Design review of the part built by this model. Coordinates are the model's own, in mm. A direction names the side the tool comes from. Round coordinates to 2 decimals unless told otherwise and drop trailing zeros. Order: outer loops, then holes, each group sorted by start corner. A loop starts at its lowest first (then second) coordinate and runs counter-clockwise, first axis right, second up. Notation, with made-up numbers: (58.5, -3) - (109.5, -3) arc R6 cw to (109.5, 8) - close; hole circle Ø3 at (54, 48.25). An arc over 180 degrees is marked (long way). Answer as a JSON object with one key per item and string values. Group by question number.
Autodesk Inventor part; units mm, degrees
ref_plane "YZ Plane" through (0, 0, 0) normal (1, 0, 0) x (0, 1, 0)
ref_plane "XZ Plane" through (0, 0, 0) normal (0, 1, 0) x (-1, 0, 0)
ref_plane "XY Plane" through (0, 0, 0) normal (0, 0, 1) x (1, 0, 0)
sketch "Sketch1" plane through (0, 0, 0) normal (1, 0, 0) x (0, 1, 0)
  line L0 (0, 0) -> (21.59, 0)
  line L1 (21.59, 0) -> (21.59, -120.8278)
  line L2 (21.59, -120.8278) -> (0, -120.8278)
  line L3 (0, -120.8278) -> (0, 0)
  dimension "d0" = 21.59
  dimension "d1" = 120.8278
extrude "Extrusion1" add sketch "Sketch1" along normal blind 4.7625
sketch "Sketch2" plane through (0, 21.59, 0) normal (0, 1, 0) x (1, 0, 0)
  line L0 (0, 0) -> (-3.2071, -18.1884)
  line L1 (0, 0) -> (18.469, 0) construction
  line L2 (0, 0) -> (13.0579, -2.3025)
  line L3 (0, 0) -> (13.2594, 0) construction
  dimension "d4" = 100
  dimension "d24" = 10
ref_plane "Work Plane1" through (0, 21.59, 0) normal (-0.9848078, 0, -0.1736482) x (-0.1736482, 0, 0.9848078)
sketch "Sketch3" plane through (0, 21.59, 0) normal (-0.9848078, 0, -0.1736482) x (-0.1736482, 0, 0.9848078)
  line L0 (-0.827, 0) -> (-0.827, -21.59)
  line L1 (-0.827, -21.59) -> (-119.8192, -21.59)
  line L2 (-119.8192, -21.59) -> (-119.8192, 0)
  line L3 (-119.8192, 0) -> (-0.827, 0)
  line L4 (0, -21.59) -> (0, 0)
  line L5 (0, -21.59) -> (-0.827, -21.59)
  line L6 (-0.827, 0) -> (-0.827, -21.59)
  line L7 (0, 0) -> (-0.827, 0)
  line L8 (0, -21.59) -> (0, 0)
  circle A0 centre (-0.8636, -10.795) radius 9.525
  dimension "d6" = 21.59
  dimension "d50" = 19.05
  dimension "d51" = 0.8636
extrude "Extrusion2" add sketch "Sketch3" against normal blind 4.7625 contours A0 L4 L0 | L0 A0 | A0 L4
ref_plane "Work Plane3" through (0, 0, 0) normal (-0.1736482, 0, 0.9848078) x (0, 1, 0)
sketch "Sketch9" plane through (4.7625, 0, 0) normal (1, 0, 0) x (0, 0, -1)
  line L0 (0, 21.59) -> (0, 20.3199)
  line L1 (0, 0) -> (120.8278, 0)
  line L2 (120.8278, 0) -> (120.8278, 21.59)
  line L3 (120.8278, 21.59) -> (0, 21.59)
  circle A0 centre (109.6528, 10.795) radius 8
  line L4 (102.7246, 14.795) -> (116.581, 14.795)
  line L5 (116.581, 14.795) -> (116.581, 6.795)
  line L6 (116.581, 6.795) -> (102.7246, 6.795)
  line L7 (102.7246, 6.795) -> (102.7246, 14.795)
  ellipse E0 centre (0.0372, 10.795) end of major axis (9.7091, 10.795) minor radius 9.525 (0, 1.2701) -> (0, 20.3199) ccw
  line L8 (0, 1.2701) -> (0, 0)
  dimension "d34" = 16
  dimension "d35" = 8
  dimension "d36" = 4
  dimension "d37" = 21.59
  dimension "d38" = 10.795
  dimension "d39" = 11.175
hole "Hole3" at (4.7625, 14.795, -102.7246) at (4.7625, 6.795, -102.7246) at (4.7625, 14.795, -116.581) at (4.7625, 6.795, -116.581) direction (-1, 0, 0) diameter 2.794 end through all
sketch "Sketch11" plane through (4.8401, 10.795, -0.0235) normal (0.9848078, 0, 0.1736482) x (0.1736482, 0, -0.9848078)
  circle A0 centre (0, 0) radius 9.525
  point P0 (-0.8636, -10.795)
hole "Hole4" at (4.8401, 10.795, -0.0235) direction (-0.9848078, 0, -0.1736482) diameter 12.827 end through all
sketch "Sketch12" plane through (4.8401, 10.795, -0.0235) normal (0.9848078, 0, 0.1736482) x (0.1736482, 0, -0.9848078)
  circle A0 centre (0, 0) radius 6.4135
  circle A1 centre (0, 0) radius 9.525
  ellipse E0 centre (114.7733, 4) end of major axis (114.7733, 2.603) minor radius 1.3758
  ellipse E1 centre (101.1274, 4) end of major axis (101.1274, 2.603) minor radius 1.3758
  ellipse E2 centre (101.1274, -4) end of major axis (101.1274, -5.397) minor radius 1.3758
  ellipse E3 centre (114.7733, -4) end of major axis (114.7733, -5.397) minor radius 1.3758
  arc A2 (-0.0366, -9.5249) -> (-0.0366, 9.5249) centre (0, 0) ccw
  line L0 (-0.0366, -9.5249) -> (-0.0366, -10.795)
  line L1 (-0.0366, -10.795) -> (118.9556, -10.795)
  line L2 (118.9556, -10.795) -> (118.9556, 10.795)
  line L3 (118.9556, 10.795) -> (-0.0366, 10.795)
  line L4 (-0.0366, 10.795) -> (-0.0366, 9.5249)
  line L5 (-0.0366, -6.4134) -> (4.7259, -6.4134)
  line L6 (4.7259, -6.4134) -> (4.7259, -29.9338)
  line L7 (4.7259, -29.9338) -> (-0.0366, -29.9338)
  line L8 (-0.0366, -29.9338) -> (-0.0366, -6.4134)
  point P0 (-0.8636, -10.795)
  dimension "d59" = 4.7625
  dimension "d60" = 23.5204
extrude "Extrusion5" add sketch "Sketch12" against normal blind 4.7625 contours L5 L6 A1 L8 | A1 L6 L1 L0 | L1 L6 L7 L8 picked at (2.6364, -7.2637)
equation "\"d36\" = 0.5 * d35"
equation "\"d38\" = 0.5 * d37"
properties part number "WheelIntakeMotorMount2.0"
1. Mouldability with a two-part tool opening along Z and no side actions: class faces 4 (the flat face through (2, 11, -120.828)), 5 (the flat face through (2.5, -9.1, -0.4)), 6 (the cylindrical face through (1.33, 10.73, 9.03)), 7 (the cylindrical face through (2.348, 14.375, -117.913)) as pulls with the +Z half, pulls with the -Z half, needs draft (parallel to the pull), parting line crosses it, or undercut.
2. Take a section at A-A, the plane z = -46.5. Give the boundary of the cut face in (x, y).
3. Tool access review of faces 1 (the cylindrical face through (2.35, 6.73, -101.33)), 2 (the flat face through (0.55, -9.44, -3.13)), 3 (the flat face through (0, 11, -60)): name each direction out of +Z, -Z, +X, -X, +Y, -Y from which nothing blocks a thin tool from reaching the whole face with its end or side.
4. Take a section at B-B, the plane y = -5.5. Give the boundary of the cut face in (x, z).
5. Clearance check with flat-ended pins moving along their axes: P1, Ø4.5, axis at y = 6.8, z = -102.72, coming from the -X side; P2, Ø6.5, axis at y = 12.5, z = -44, coming from the +X side; P3, Ø2.5, axis at x = 2.5, z = -44.5, coming from the -Y side. State where each tip first meets the part, or that it passes through.
6. To check wall thickness, follow line 1 (Y direction, x = 2.25, z = -102.5); line 2 (Z direction, x = 3.25, y = 16); line 3 (Y direction, x = 0.25, z = -7.5). State the ranges of each line that lie inside material, in increasing order. Write a range as from..to.
Response values:
{
 "1": {"face 4": "pulls with the -Z half", "face 5": "pulls with the +Z half", "face 6": "parting line crosses it", "face 7": "undercut"},
 "2": {"outline": "(0, 0) - (4.76, 0) - (4.76, 21.59) - (0, 21.59) - close"},
 "3": {"face 1": "+X, -X", "face 2": "-Z, -X, -Y", "face 3": "-Z, -X, +Y, -Y"},
 "4": {"outline": "(0.14, -0.81) - (0.97, -5.5) - (5.66, -4.68) - (4.83, 0.01) - close"},
 "5": {"P1": "x = 0", "P2": "x = 4.76", "P3": "y = 0"},
 "6": {"line 1": "0..5.42, 8.17..13.42, 16.17..21.59", "line 2": "-120.83..-117.29, -115.87..-103.43, -102.02..-4.11, 3.5..7.8", "line 3": "0..21.59"}
}
